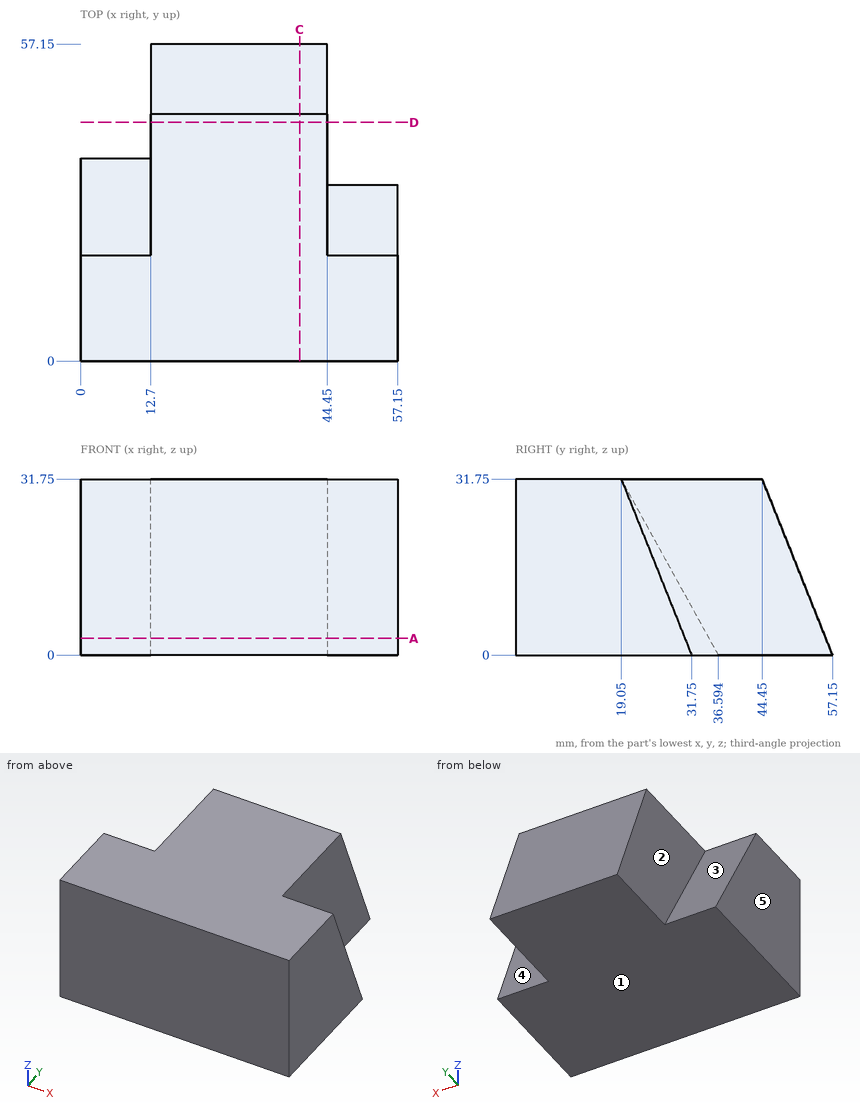
Source: three-view drawing plus pictorial views. Frame: mm from the lowest corner of the part. A direction names the side the tool comes from. Round coordinates to 2 decimals unless told otherwise and drop trailing zeros. Loops run counter-clockwise (first coordinate to the right, second up) from the corner with the lowest first, then second, coordinate; pieces in that order, holes last.
Q1. Ray query, line 1 (X direction, y = 24, z = 24); line 2 (Y direction, x = 24.5, z = 17.5); line 3 (Y direction, x = 19, z = 22.5). Return the intervals inside material, ascending.
Q2. First-contact query: P1, Ø8, axis at y = 36.5, z = 11.5, coming from the -X side; P2, Ø3, axis at x = 7.5, y = 29.5, coming from the +Z side; P3, Ø9.5, axis at y = 47, z = 19.5, coming from the +X side. Flat tips, straight axial feed; report the tip coordinate or a pass-through.
Q3. Mould query, pull axis Z, two halves, no side actions, for the marked faces 1, 2 and 3. Classes: pulls with the +Z half, pulls with the -Z half, needs draft (parallel to the pull), parting line crosses it, or undercut.
Q4. Section D-D, the plane y = 43. Return loops of the section in (x, z), plus the area to 3 significant figures.
Q5. Section C-C, the plane x = 39.5. Return loops of the section in (y, z), plus the area to 3 significant figures.
Q6. Access query for the marked faces 4 and 5. Directions: +Z, -Z, +X, -X, +Y, -Y. A direction counts if a zero-diameter tool reaches every point of the face in a straight line with its end or side. Return the directions, or none.
Q7. Section A-A, the plane z = 3. Return loops of the section in (x, y), plus the area to 3 significant figures.
Solutions:
1. line 1: x = 12.7 to 44.45
1. line 2: y = 0 to 50.15
1. line 3: y = 0 to 48.15
2. P1: stops at x = 12.7
2. P2: stops at z = 15.55
2. P3: stops at x = 44.45
3. face 1: pulls with the -Z half
3. face 2: needs draft
3. face 3: pulls with the +Z half
4. outline: (12.7, 0) - (44.45, 0) - (44.45, 31.75) - (12.7, 31.75) - close
4. area: 1,010 mm2
5. outline: (0, 0) - (57.15, 0) - (44.45, 31.75) - (0, 31.75) - close
5. area: 1,610 mm2
6. face 4: +Z, +X, +Y
6. face 5: +Z, -Z, -X, +Y, -Y
7. outline: (0, 0) - (57.15, 0) - (57.15, 30.55) - (44.45, 30.55) - (44.45, 55.95) - (12.7, 55.95) - (12.7, 34.94) - (0, 34.94) - close
7. area: 2,610 mm2
